Can you work these out from the model? Positions are in its coordinate system, mm. Give positions to 0.01 mm unless a question says otherwise; leave off trailing zeros. Loops run counter-clockwise (first coordinate to the right, second up) from the corner with the lowest first, then second, coordinate; pieces in that order, holes last. Notation, with made-up numbers: (75, 23.5) - (82, 23.5) arc R20 ccw to (82, 62.5) - close; hole circle Ø4 at (87, 45.5). An arc over 180 degrees is marked (long way). Answer in a Markdown table with one row per item.
from build123d import *

# Parameters (mm, degrees)
SKETCH_1_R      = 2.5
SKETCH_1_R_2    = 2
EXTRUDE_1_DEPTH = 5


with BuildPart() as part:
    # 草图1 → 凸台-拉伸1 (new body)
    with BuildSketch(Plane.XY):
        with BuildLine():
            Line((5, 0), (295, 0))
            ThreePointArc((295, 0), (298.535533906, 1.464466094), (300, 5))
            Line((300, 5), (300, 295))
            ThreePointArc((300, 295), (298.535533906, 298.535533906), (295, 300))
            Line((295, 300), (5, 300))
            ThreePointArc((5, 300), (1.464466094, 298.535533906), (0, 295))
            Line((0, 295), (0, 245))
            ThreePointArc((0, 245), (1.464466094, 241.464466094), (5, 240))
            Line((5, 240), (60, 240))
            ThreePointArc((60, 240), (150, 150), (60, 60))
            Line((60, 60), (5, 60))
            ThreePointArc((5, 60), (1.464466094, 58.535533906), (0, 55))
            Line((0, 55), (0, 5))
            ThreePointArc((0, 5), (1.464466094, 1.464466094), (5, 0))
        make_face()
        with Locations((10, 250)):
            Circle(SKETCH_1_R, mode=Mode.SUBTRACT)
        with Locations(Location((290, 250, 0), (0, 0, 180))):
            Circle(SKETCH_1_R, mode=Mode.SUBTRACT)
        with Locations(Location((10, 50, 0), (0, 0, 180))):
            Circle(SKETCH_1_R, mode=Mode.SUBTRACT)
        with Locations((290, 50)):
            Circle(SKETCH_1_R, mode=Mode.SUBTRACT)
        with Locations((8, 292)):
            Circle(SKETCH_1_R_2, mode=Mode.SUBTRACT)
        with Locations((69, 292)):
            Circle(SKETCH_1_R_2, mode=Mode.SUBTRACT)
        with Locations((69, 261)):
            Circle(SKETCH_1_R_2, mode=Mode.SUBTRACT)
        with Locations((8, 261)):
            Circle(SKETCH_1_R_2, mode=Mode.SUBTRACT)
        with Locations(Location((8, 39, 0), (0, 0, 180))):
            Circle(SKETCH_1_R_2, mode=Mode.SUBTRACT)
        with Locations(Location((69, 39, 0), (0, 0, 180))):
            Circle(SKETCH_1_R_2, mode=Mode.SUBTRACT)
        with Locations(Location((69, 8, 0), (0, 0, 180))):
            Circle(SKETCH_1_R_2, mode=Mode.SUBTRACT)
        with Locations(Location((8, 8, 0), (0, 0, 180))):
            Circle(SKETCH_1_R_2, mode=Mode.SUBTRACT)
        with Locations((200, 220)):
            Circle(SKETCH_1_R_2, mode=Mode.SUBTRACT)
        with Locations((240, 220)):
            Circle(SKETCH_1_R_2, mode=Mode.SUBTRACT)
        with Locations((180, 115)):
            Circle(SKETCH_1_R_2, mode=Mode.SUBTRACT)
        with Locations((260, 35)):
            Circle(SKETCH_1_R_2, mode=Mode.SUBTRACT)
    extrude(amount=EXTRUDE_1_DEPTH)


solid = part.part
Q1. If I drill on line 1 (Y direction, x = 290, z = 1.05); line 2 (X direction, y = 48, z = 2.55); line 3 (X direction, y = 220, z = 2.1), over which ranges is the centre line in solid material (lowest first)? Write a range as [from, to].
Checked values:
| item | result |
|---|---|
| line 1 | y = [0, 47.5], [52.5, 247.5], [252.5, 300] |
| line 2 | x = [0, 8.5], [11.5, 288.5], [291.5, 300] |
| line 3 | x = [116.57, 198], [202, 238], [242, 300] |
Q2. Imagine slicing it at B-B, the plane z = 2.95. Count the separate pieces of the cut face and the enclosed holes in it, and give its area (3 significant figures).
Checked values:
| item | result |
|---|---|
| separate pieces | 1 |
| enclosed holes | 16 |
| area | 66,200 mm² |
Q3. Imagine slicing it at A-A, the plane x = 45.5. Write out the boundary of the cut face in (y, z).
Checked values:
| item | result |
|---|---|
| outline | (0, 0) - (60, 0) - (60, 5) - (0, 5) - close; (240, 0) - (300, 0) - (300, 5) - (240, 5) - close |
Q4. Imagine slicing it at D-D, the plane y = 191.5. Write out the boundary of the cut face in (x, z), and give its area (3 significant figures).
Checked values:
| item | result |
|---|---|
| outline | (139.86, 0) - (300, 0) - (300, 5) - (139.86, 5) - close |
| area | 801 mm² |
Q5. If we mould it in two halves opening along Y, with no side actions, what happens to faces 1 (the face through (181, 152, 5)), 2 (the face through (149.98, 151.98, 2.46))? For each: released by +Y, released by -Y, zero draft, split by the parting line, or undercut.
Checked values:
| item | result |
|---|---|
| face 1 | zero draft |
| face 2 | undercut |
Q6. Imagine slicing it at C-C, the plane y = 150. Write out the boundary of the cut face in (x, z).
Checked values:
| item | result |
|---|---|
| outline | (150, 0) - (300, 0) - (300, 5) - (150, 5) - close |
Q7. For pin 1 (1 mm diameter, centred on y = 218, z = 3, fed in from -X); pin 2 (4.5 mm diameter, centred on x = 69, y = 8, fed in from -Z), each with a flat end and sliding along its axis, tell me the tip position at first contact or that it passes through.
Checked values:
| item | result |
|---|---|
| pin 1 | stops at x = 118.38 |
| pin 2 | stops at z = 0 |
